Part model, mm, in its own coordinate system. A direction names the side the tool comes from. Coordinates: 2 decimals unless noted, no trailing zeros. Order: outer loops, then holes, each group sorted by start corner. A loop starts at its lowest first (then second) coordinate and runs counter-clockwise, first axis right, second up. Notation, with made-up numbers: M 63.5,-24 L 85.5,-24 A14 cw 85.5,-1 Z; hole C 17,-13 d4. An arc over 180 degrees is marked long. Answer in a Markdown table with one row per item. Add a question column.
from build123d import *

# Parameters (mm, degrees)
F0_R     = 12.5
F1_DEPTH = 120
F2_SIZE  = 1
F3_R     = 17.5
F4_DEPTH = 10


with BuildPart() as f1:
    # F0 (on Front) → F1 (new body)
    with BuildSketch(Plane.XZ):
        Circle(F0_R)
    extrude(amount=F1_DEPTH)

    # F2
    f2_edges = [f1.edges().sort_by_distance(p)[0] for p in [
        (-12.5, -120, 0),
        (-12.5, 0, 0),
    ]]
    chamfer(f2_edges, length=F2_SIZE)

    # F3 (on Front) → F4 (join)
    with BuildSketch(Plane.XZ):
        Circle(F3_R)
    extrude(amount=F4_DEPTH)


solid = f1.part
(1) Slice it at D-D (z = -15). List the corners of the cut face in (x, y).
(2) Drop flat-ended pins along their axis: P1, Ø4, axis at x = 10.5, y = -45.5, coming from the +Z side; P2, Ø1, axis at x = 8, y = -60.5, coming from the +Z side; P3, Ø8, axis at x = -6.5, y = -48, coming from the -Z side. Give the stop position or say it passes through.
(3) Slice it at C-C (y = -69.5). List the corners of the cut face in (x, z).
(4) Slice it at A-A (x = 0). List the corners of the cut face in (y, z), and give its area (3 significant figures).
(5) Slice it at B-B (z = 0). List the corners of the cut face in (x, y), and give its area (3 significant figures).
(6) Wall check: line 1 (Z direction, x = 0.5, y = -57); line 2 (Y direction, x = 7, z = -12); line 3 (X direction, y = -40, z = 10). Give the ranges that are in metal, low to high.
(7) 3-axis set-ups, long thin cutter, end or side, ignore diameter. For faces 1 (the flat face through (8, -10, -11)), 2 (the flat face through (0, -120, 0)): which of +Z, -Z, +X, -X, +Y, -Y reach the whole face in a straight line?
Computed:
| question | item | result |
|---|---|---|
| 1 | outline | M -9.01,-10 L 9.01,-10 L 9.01,0 L -9.01,0 Z |
| 2 | P1 | stops at z = 9.17 |
| 2 | P2 | stops at z = 10 |
| 2 | P3 | stops at z = -12.25 |
| 3 | outline | C 0,0 d25 |
| 4 | outline | M -120,-11.5 L -119,-12.5 L -10,-12.5 L -10,-17.5 L 0,-17.5 L 0,17.5 L -10,17.5 L -10,12.5 L -119,12.5 L -120,11.5 Z |
| 4 | area | 3,100 mm^2 |
| 5 | outline | M -17.5,-10 L -12.5,-10 L -12.5,-119 L -11.5,-120 L 11.5,-120 L 12.5,-119 L 12.5,-10 L 17.5,-10 L 17.5,0 L -17.5,0 Z |
| 5 | area | 3,100 mm^2 |
| 6 | line 1 | z = -12.49 to 12.49 |
| 6 | line 2 | y = -10 to 0 |
| 6 | line 3 | x = -7.5 to 7.5 |
| 7 | face 1 | -Y |
| 7 | face 2 | +Z, -Z, +X, -X, -Y |
